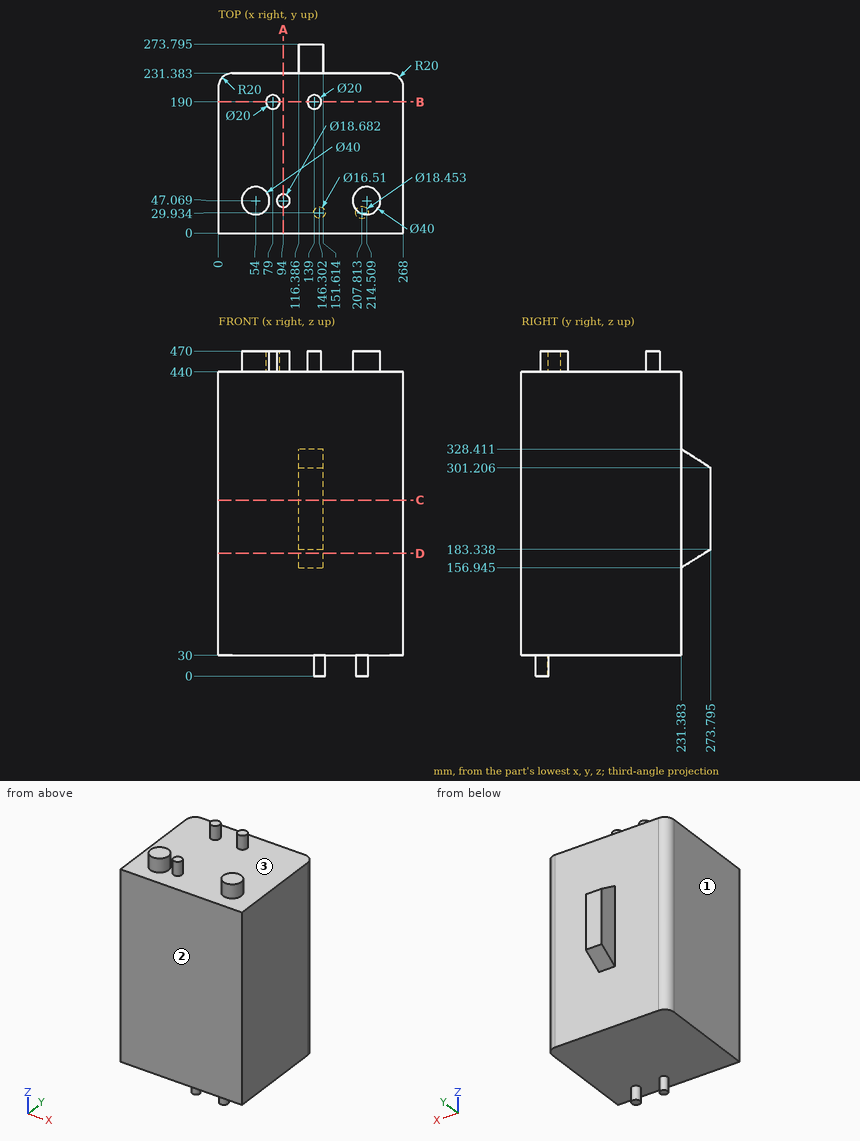
Design review of the part shown in the three views and the two pictorial views. Dimensions are in mm from the part's minimum x, y and z. Round coordinates to 2 decimals unless told otherwise and drop trailing zeros. Order: outer loops, then holes, each group sorted by start corner. A loop starts at its lowest first (then second) coordinate and runs counter-clockwise, first axis right, second up.
Q1. Mouldability with a two-part tool opening along X and no side actions: class the marked faces 1, 2 and 3 as pulls with the +X half, pulls with the -X half, needs draft (parallel to the pull), parting line crosses it, or undercut.
Findings below:
face 1: pulls with the -X half
face 2: needs draft
face 3: undercut
Q2. Insertion check: P1, Ø21, axis at y = 262.5, z = 224.5, coming from the +X side; P2, Ø12, axis at x = 136.5, y = 151.5, coming from the +Z side; P3, Ø21, axis at y = 261, z = 225, coming from the -X side. Each pin has a flat end and moves straight along its axis. Give the tip position at first contact, or say it passes through.
Findings below:
P1: stops at x = 151.61
P2: stops at z = 440
P3: stops at x = 116.39
Q3. Wall thickness on line 1 (Z direction, x = 47, y = 192.5); line 2 (Y direction, x = 78, z = 303); line 3 (Z direction, x = 121.5, y = 256.5) (1 decimal): over which ranges is each line inside the solid? List them lowest first.
Findings below:
line 1: z = 30 to 440
line 2: y = 0 to 231.38
line 3: z = 172.6 to 312.3
Q4. We need section A-A, the plane x = 94. Give the boundary of the cut face in (y, z), plus the area to 3 significant figures.
Findings below:
outline: (0, 30) - (231.38, 30) - (231.38, 440) - (56.41, 440) - (56.41, 470) - (37.73, 470) - (37.73, 440) - (0, 440) - close
area: 95,400 mm2
Q5. We need section B-B, the plane y = 190. Give the boundary of the cut face in (x, z), plus the area to 3 significant figures.
Findings below:
outline: (0, 30) - (268, 30) - (268, 440) - (149, 440) - (149, 470) - (129, 470) - (129, 440) - (89, 440) - (89, 470) - (69, 470) - (69, 440) - (0, 440) - close
area: 111,000 mm2
Q6. We need section D-D, the plane z = 177.5. Give the boundary of the cut face in (x, y), plus the area to 3 significant figures.
Findings below:
outline: (0, 0) - (268, 0) - (268, 211.38) arc R20 ccw to (248, 231.38) - (151.61, 231.38) - (151.61, 264.41) - (116.39, 264.41) - (116.39, 231.38) - (20, 231.38) arc R20 ccw to (0, 211.38) - close
area: 63,000 mm2
Q7. We need section C-C, the plane z = 254.5. Give the boundary of the cut face in (x, y) (1 decimal), plus the area to 3 significant figures.
Findings below:
outline: (0, 0) - (268, 0) - (268, 211.4) arc R20 ccw to (248, 231.4) - (151.6, 231.4) - (151.6, 273.8) - (116.4, 273.8) - (116.4, 231.4) - (20, 231.4) arc R20 ccw to (0, 211.4) - close
area: 63,300 mm2
